Check sheet for the drawn part. Datum: minimum x, y, z corner. Units: mm. A direction names the side the tool comes from. Give positions to 0.01 mm unless a question says otherwise; leave off trailing zeros. Write each loop counter-clockwise with the first axis right and the second up, starting at its lowest first coordinate (ties: lowest second). Pieces come first, ordered by that corner, then holes. Notation, with made-up numbers: M 67,-23 L 123,-23 A17 ccw 123,6 Z; hole C 19.5,-38.5 d1. An arc over 180 degrees is marked long. Use CSV: the item, a comma, the result in double quotes. Start each with the question number.
1. Cross-section at A-A, the plane z = 11. Enter the section's corners in (x, y).
2. Scan lines: line 1 (Z direction, x = 10, y = 2.95); line 2 (Z direction, x = 14.25, y = 8); line 3 (X direction, y = 3, z = 11). Record each from-to range of solid material in increasing order.
3. Mould release check, pull along Z, two halves, no side actions. Record for the marked faces 1, 2, 3 and 4: +Z half, -Z half, draft (parallel to the pull), parting line (faces both ways), or undercut.
4. Cross-section at D-D, the plane y = 34.5. Enter the section's corners in (x, z), and give its area (3 significant figures).
5. Cross-section at C-C, the plane x = 10. Enter the section's corners in (y, z).
6. Depth check by flat-ended pin: P1, Ø6, axis at x = 11.5, z = 30, coming from the +Y side; P2, Ø5, axis at x = 10, z = 39, coming from the +Y side; P3, Ø4, axis at y = 27.5, z = 1.5, coming from the -X side; P4, Ø5.5, axis at y = 20, z = 2.5, coming from the +X side. Enter the tip coordinate at first touch or a pass-through.
7. Cross-section at B-B, the plane y = 47. Enter the section's corners in (x, z), and give its area (3 significant figures).
8. Access from +Z, -Z, +X, -X, +Y, -Y to the whole of each face (thin tool, end or side, straight path). Record for the marked faces 5 and 6.
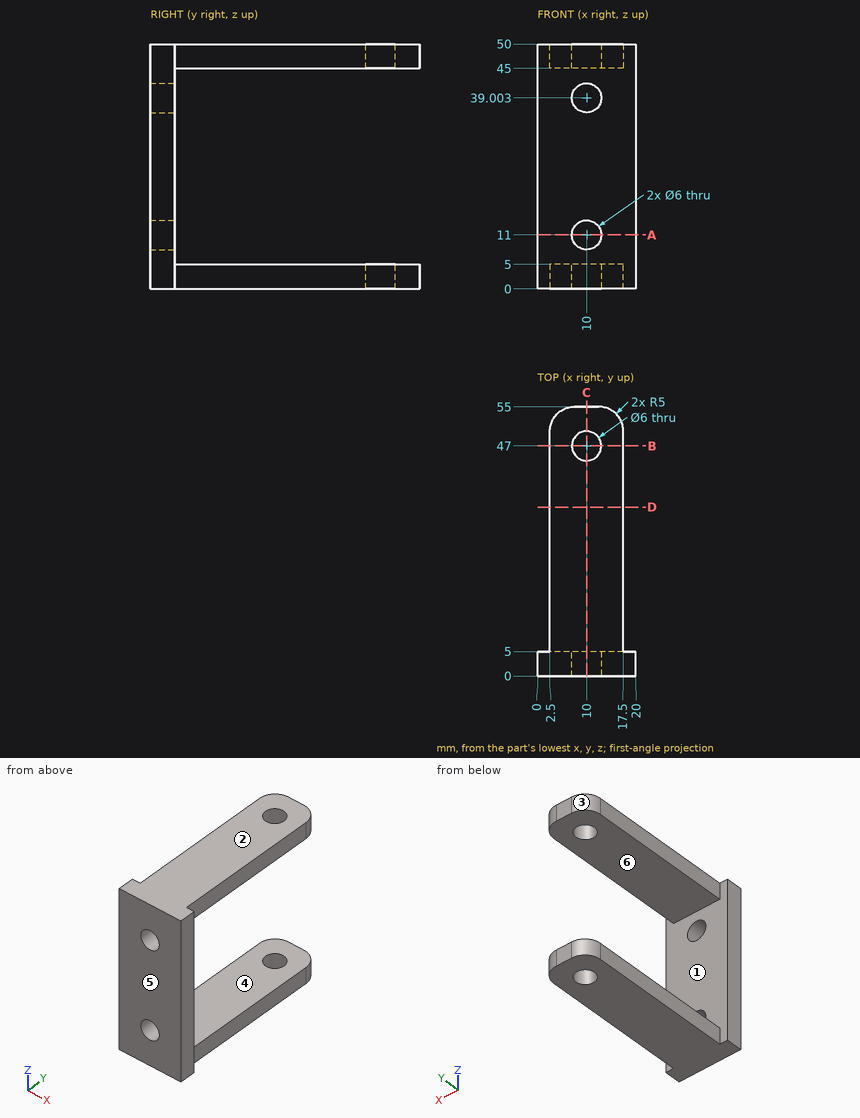
Worked answers:
1,outline,"M 0,0 L 7,0 L 7,5 L 0,5 Z; M 13,0 L 20,0 L 20,5 L 13,5 Z"
2,line 1,"z = 0 to 8, 14 to 36, 42 to 50"
2,line 2,"z = 0 to 5, 45 to 50"
2,line 3,"x = 0 to 7, 13 to 20"
3,face 1,"undercut"
3,face 2,"+Z half"
3,face 3,"draft"
3,face 4,"undercut"
4,outline,"M 2.5,0 L 17.5,0 L 17.5,5 L 2.5,5 Z; M 2.5,45 L 17.5,45 L 17.5,50 L 2.5,50 Z"
4,area,"150 mm^2"
5,outline,"M 0,0 L 44,0 L 44,5 L 5,5 L 5,8 L 0,8 Z; M 0,14 L 5,14 L 5,36 L 0,36 Z; M 0,42 L 5,42 L 5,45 L 44,45 L 44,50 L 0,50 Z; M 50,0 L 55,0 L 55,5 L 50,5 Z; M 50,45 L 55,45 L 55,50 L 50,50 Z"
6,P1,"stops at y = 5"
6,P2,"passes through"
6,P3,"stops at x = 2.5"
6,P4,"stops at x = 17.5"
7,outline,"M 2.5,0 L 7,0 L 7,5 L 2.5,5 Z; M 2.5,45 L 7,45 L 7,50 L 2.5,50 Z; M 13,0 L 17.5,0 L 17.5,5 L 13,5 Z; M 13,45 L 17.5,45 L 17.5,50 L 13,50 Z"
7,area,"90.0 mm^2"
8,face 5,"+Z, -Z, +X, -X, -Y"
8,face 6,"+X, -X, +Y"
